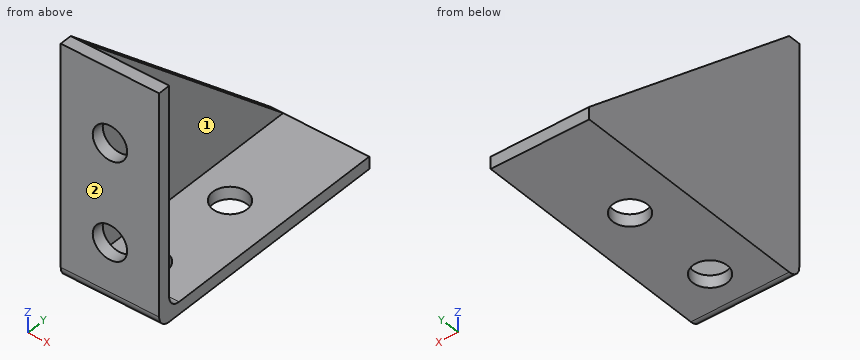
```python
from build123d import *

# Parameters (mm, degrees)
CROQUIS1_W              = 40
CROQUIS1_H              = 105
SALIENTE_EXTRUIR1_DEPTH = 5
CROQUIS2_R              = 7
CORTAR_EXTRUIR1_DEPTH   = 5
CROQUIS2_3_R            = 7
CORTAR_EXTRUIR2_DEPTH   = 5
CROQUIS4_W              = 40
CROQUIS4_H              = 5
SALIENTE_EXTRUIR2_DEPTH = 90
CROQUIS5_R              = 7
CORTAR_EXTRUIR3_DEPTH   = 90
CROQUIS5_3_R            = 7
CORTAR_EXTRUIR4_DEPTH   = 90
REDONDEO3_R             = 5
REDONDEO4_R             = 5
SALIENTE_EXTRUIR3_START = -5
SALIENTE_EXTRUIR3_DEPTH = 5


with BuildPart() as part:
    # Croquis1 → Saliente-Extruir1 (new body)
    with BuildSketch(Plane.XY):
        with Locations((20, 52.5)):
            Rectangle(CROQUIS1_W, CROQUIS1_H)
    extrude(amount=SALIENTE_EXTRUIR1_DEPTH)

    # Croquis2 → Cortar-Extruir1 (cut)
    with BuildSketch(Plane.XY.offset(5)):
        with Locations((20, 60)):
            Circle(CROQUIS2_R)
    extrude(amount=-CORTAR_EXTRUIR1_DEPTH, mode=Mode.SUBTRACT)

    # Croquis2_3 → Cortar-Extruir2 (cut)
    with BuildSketch(Plane.XY.offset(5)):
        with Locations((20, 20)):
            Circle(CROQUIS2_3_R)
    extrude(amount=-CORTAR_EXTRUIR2_DEPTH, mode=Mode.SUBTRACT)

    # Croquis4 → Saliente-Extruir2 (add)
    with BuildSketch(Plane.XY.offset(5)):
        with Locations((20, 2.5)):
            Rectangle(CROQUIS4_W, CROQUIS4_H)
    extrude(amount=SALIENTE_EXTRUIR2_DEPTH)

    # Croquis5 → Cortar-Extruir3 (cut)
    with BuildSketch(Plane(origin=(0, 5, 0), x_dir=(1, 0, 0), z_dir=(0, 1, 0))):
        with Locations(Location((20, -25, 0), (0, 0, 270))):
            Circle(CROQUIS5_R)
    extrude(amount=-CORTAR_EXTRUIR3_DEPTH, mode=Mode.SUBTRACT)

    # Croquis5_3 → Cortar-Extruir4 (cut)
    with BuildSketch(Plane(origin=(0, 5, 0), x_dir=(1, 0, 0), z_dir=(0, 1, 0))):
        with Locations(Location((20, -25, 0), (0, 0, 270))):
            Circle(CROQUIS5_3_R)
        with Locations(Location((20, -65, 0), (0, 0, 270))):
            Circle(CROQUIS5_3_R)
    extrude(amount=-CORTAR_EXTRUIR4_DEPTH, mode=Mode.SUBTRACT)

    # Redondeo3
    redondeo3_edges = [part.edges().sort_by_distance(p)[0] for p in [
        (20, 5, 5),
    ]]
    fillet(redondeo3_edges, radius=REDONDEO3_R)

    # Redondeo4
    redondeo4_edges = [part.edges().sort_by_distance(p)[0] for p in [
        (20, 0, 0),
    ]]
    fillet(redondeo4_edges, radius=REDONDEO4_R)

    # Croquis6 → Saliente-Extruir3 (add)
    with BuildSketch(Plane.ZY.offset(SALIENTE_EXTRUIR3_START)):
        with BuildLine():
            Line((5, 105), (95, 5))
            Line((95, 5), (10, 5))
            ThreePointArc((10, 5), (6.464466094, 6.464466094), (5, 10))
            Line((5, 10), (5, 105))
        make_face()
    extrude(amount=SALIENTE_EXTRUIR3_DEPTH)


solid = part.part
```
CAD build for the part. Positions are in the model's coordinates, mm. Face numbers are marked on the shaded views. A direction names the side the tool comes from. Round coordinates to 2 decimals unless told otherwise and drop trailing zeros. Write each loop counter-clockwise with the first axis right and the second up, starting at its lowest first coordinate (ties: lowest second). Pieces come first, ordered by that corner, then holes. Notation, with made-up numbers: (-34, 6) -> (17, 6) arc R16 ccw to (17, 14) -> close; hole circle Ø8 at (29.25, 41.5). An arc over 180 degrees is marked (long way). Answer in a Markdown table with one row per item. Add a question column.
Item 1: Drop flat-ended pins along their axis: pin 1 Ø8 at (x, y) = (33.5, 70) entering from +Z; pin 2 Ø12 at (x, z) = (4.5, 30.5) entering from +Y; pin 3 Ø3 at (y, z) = (60.5, 30.5) entering from +X. Give the stop position or say it passes through.
Item 2: Saw through at B-B, the plane x = 20. Write the cut outline in (y, z).
Item 3: Saw through at D-D, the plane x = 9. Write the cut outline in (y, z), then the cut area to 3 significant figures.
Item 4: Drill centre lines: line 1 (X direction, y = 2, z = 25); line 2 (Y direction, x = 20, z = 3.25); line 3 (Z direction, x = 8, y = 11.5). Where is each one in solid material? Low to high. Write a range as from..to.
Item 5: Which spindle directions (+Z, -Z, +X, -X, +Y, -Y) get a long thin tool onto all of the face, cutting with end or side? Do the marked faces 1 and 2. Say none if no direction does.
Item 6: Saw through at A-A, the plane y = 60. Write the cut outline in (x, z).
Item 7: Saw through at C-C, the plane z = 65. Write the cut outline in (x, y).
Findings below:
| question | item | result |
|---|---|---|
| 1 | pin 1 | stops at z = 5 |
| 1 | pin 2 | stops at y = 83.33 |
| 1 | pin 3 | stops at x = 5 |
| 2 | outline | (0, 5) arc R5 ccw to (5, 0) -> (13, 0) -> (13, 5) -> (10, 5) arc R5 cw to (5, 10) -> (5, 18) -> (0, 18) -> close; (0, 32) -> (5, 32) -> (5, 58) -> (0, 58) -> close; (0, 72) -> (5, 72) -> (5, 95) -> (0, 95) -> close; (27, 0) -> (53, 0) -> (53, 5) -> (27, 5) -> close; (67, 0) -> (105, 0) -> (105, 5) -> (67, 5) -> close |
| 3 | outline | (0, 5) arc R5 ccw to (5, 0) -> (105, 0) -> (105, 5) -> (10, 5) arc R5 cw to (5, 10) -> (5, 95) -> (0, 95) -> close |
| 3 | area | 975 mm^2 |
| 4 | line 1 | x = 0..13, 27..40 |
| 4 | line 2 | y = 0.32..13, 27..53, 67..105 |
| 4 | line 3 | z = 0..5 |
| 5 | face 1 | +Z, +X, +Y |
| 5 | face 2 | +Z, -Z, +X, -X, -Y |
| 6 | outline | (0, 0) -> (13, 0) -> (13, 5) -> (5, 5) -> (5, 45.5) -> (0, 45.5) -> close; (27, 0) -> (40, 0) -> (40, 5) -> (27, 5) -> close |
| 7 | outline | (0, 0) -> (13, 0) -> (13, 5) -> (5, 5) -> (5, 38.33) -> (0, 38.33) -> close; (27, 0) -> (40, 0) -> (40, 5) -> (27, 5) -> close |
